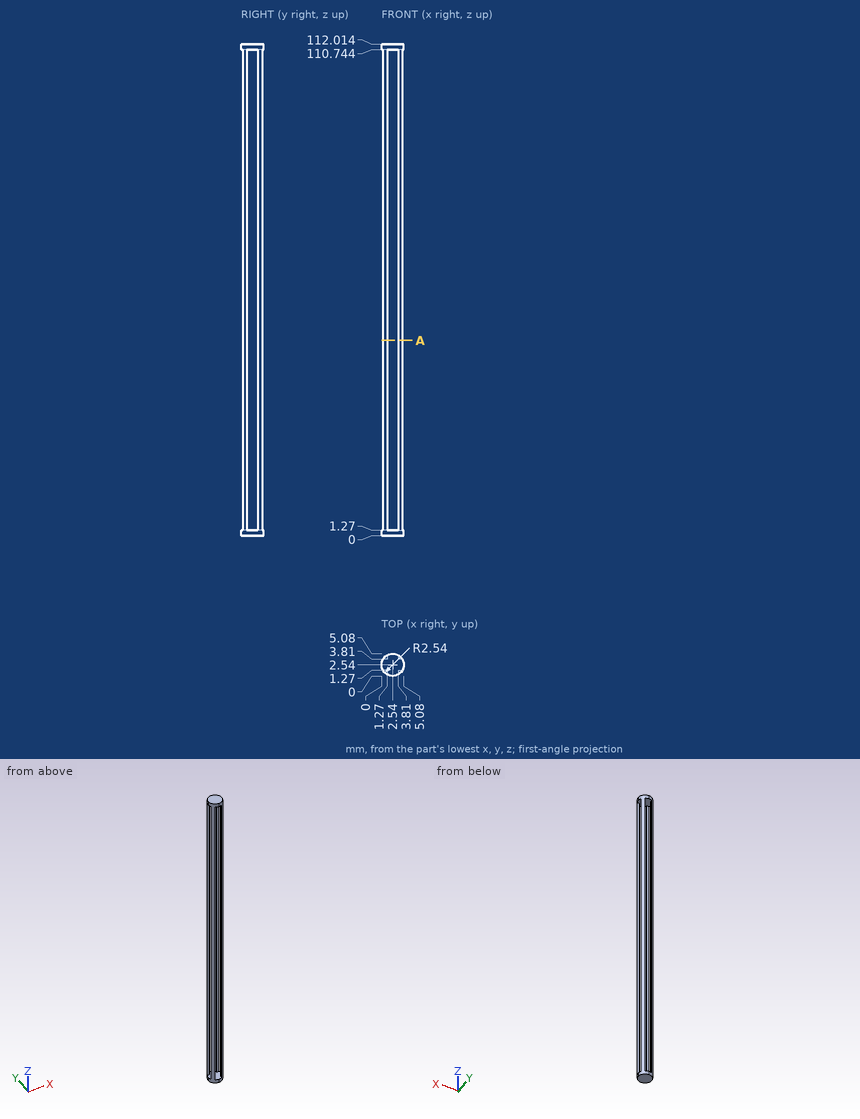
Geometry: see drawing. Coordinates: mm, zero at the bounding-box minimum. Coordinates: 2 decimals unless noted, no trailing zeros. Order: outer loops, then holes, each group sorted by start corner. A loop starts at its lowest first (then second) coordinate and runs counter-clockwise, first axis right, second up. Notation, with made-up numbers: (53, -16.5) - (80, -16.5) arc R18 cw to (80, 0.5) - close; hole circle Ø6 at (10, 44). An arc over 180 degrees is marked (long way). Write each question's results on one line, items separated by ' | '.
1) Section A-A, the plane z = 44.5. Return loops of the section in (x, y), plus the area to 3 significant figures.
Results list:
outline: (0.34, 1.27) arc R2.54 ccw to (1.27, 0.34) - (1.27, 1.27) - close; (0.34, 3.81) - (1.27, 3.81) - (1.27, 4.74) arc R2.54 ccw to start; (3.81, 0.34) arc R2.54 ccw to (4.74, 1.27) - (3.81, 1.27) - close; (3.81, 3.81) - (4.74, 3.81) arc R2.54 ccw to (3.81, 4.74) - close | area: 2.03 mm^2
2) Pin query (flat end, axial travel): pin 1 (1.5 mm diameter, centred on y = 3.5, z = 73, fed in from +X); pin 2 (1 mm diameter, centred on x = 4.5, z = 62, fed in from -Y); pin 3 (0.5 mm diameter, centred on x = 0.5, z = 64.5, fed in from +Y). Return the tip coordinate at first contact, or that it passes through.
Results list:
pin 1: x = 4.74 | pin 2: y = 0.46 | pin 3: y = 4.34
3) Line query: line 1 (Z direction, x = 2.1, y = 1.5); line 2 (X direction, y = 4.25, z = 43); line 3 (X direction, y = 1.1, z = 47). Output: solid intervals per line, ascending. Write a range as from..to.
Results list:
line 1: 0..1.27, 110.74..112.01 | line 2: 0.66..1.27, 3.81..4.42 | line 3: 0.45..1.27, 3.81..4.63
